Model file for the job. Use its own axes, mm. Face numbers are marked on the shaded views. A direction names the side the tool comes from. Round coordinates to 2 decimals unless told otherwise and drop trailing zeros. Write each loop counter-clockwise with the first axis right and the second up, starting at its lowest first coordinate (ties: lowest second). Pieces come first, ordered by that corner, then holes. Notation, with made-up numbers: (80.25, 69) - (105.25, 69) arc R26 cw to (105.25, 91) - close; hole circle Ø1 at (4.5, 71). An arc over 180 degrees is marked (long way). One line per item, written item: value.
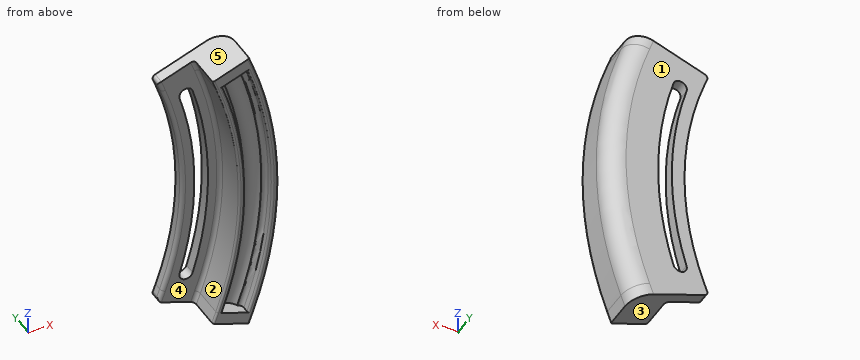
from build123d import *

# Parameters (mm, degrees)
REVOLVE_1_ANGLE     = 40
CUT_EXTRUDE_1_DEPTH = 10
FILLET_1_R          = 5
FILLET_3_R          = 1
FILLET_4_R          = 1
EXTRUDE_1_DEPTH     = 3
EXTRUDE_2_DEPTH     = 3
FILLET_6_R          = 0.5
FILLET_7_R          = 1


with BuildPart() as part:
    # 草图2 → 旋转1 (revolve, symmetric)
    with BuildSketch(Plane.XY) as revolve_1_sk:
        with BuildLine():
            Line((95, 4), (95, -5))
            Line((95, -5), (96.5, -5))
            Line((96.5, -5), (96.5, -2))
            Line((96.5, -2), (97.763932023, -2))
            ThreePointArc((97.763932023, -2), (100, -1), (102.236067977, -2))
            Line((102.236067977, -2), (103.5, -2))
            Line((103.5, -2), (103.5, -5))
            Line((103.5, -5), (105, -5))
            Line((105, -5), (105, 7))
            Line((105, 7), (85, 7))
            Line((85, 7), (85, 4))
            Line((85, 4), (95, 4))
        make_face()
    revolve(axis=Axis((0, 24.366902053, 0), (0, -1, 0)), revolution_arc=REVOLVE_1_ANGLE / 2)
    revolve(revolve_1_sk.sketch, axis=Axis((0, 24.366902053, 0), (0, 1, 0)), revolution_arc=REVOLVE_1_ANGLE / 2)

    # 草图3 → 切除-拉伸1 (cut)
    with BuildSketch(Plane(origin=(0, 7, 0), x_dir=(1, 0, 0), z_dir=(0, 1, 0))):
        with BuildLine():
            ThreePointArc((87.826997293, -26.542061834), (91.75, 1.18e-07), (87.826997225, 26.542062061))
            ThreePointArc((87.826997225, 26.542062061), (85.645571172, 27.710984674), (84.476648452, 25.529558679))
            ThreePointArc((84.476648452, 25.529558679), (88.25, 3.69e-07), (84.476648665, -25.529557973))
            ThreePointArc((84.476648665, -25.529557973), (85.645570933, -27.710984602), (87.826997293, -26.542061834))
        make_face()
    extrude(amount=-CUT_EXTRUDE_1_DEPTH, mode=Mode.SUBTRACT)

    # 圆角1
    fillet_1_edges = [part.edges().sort_by_distance(p)[0] for p in [
        (105, 7, 0),
    ]]
    fillet(fillet_1_edges, radius=FILLET_1_R)

    # 圆角3
    fillet_3_edges = [part.edges().sort_by_distance(p)[0] for p in [
        (95, 4, 0),
    ]]
    fillet(fillet_3_edges, radius=FILLET_3_R)

    # 圆角4
    fillet_4_edges = [part.edges().sort_by_distance(p)[0] for p in [
        (103.5, -2, 0),
        (96.5, -2, 0),
    ]]
    fillet(fillet_4_edges, radius=FILLET_4_R)

    # 草图5 → 凸台-拉伸1 (add)
    with BuildSketch(Plane(origin=(0, 0, 0), x_dir=(0.9396926207859081, 0, 0.34202014332566955), z_dir=(-0.34202014332566955, 0, 0.9396926207859082))):
        with BuildLine():
            Line((96.5, -5), (103.5, -5))
            Line((103.5, -5), (103.5, -3))
            ThreePointArc((103.5, -3), (103.207106781, -2.292893219), (102.5, -2))
            Line((102.5, -2), (102.236067977, -2))
            ThreePointArc((102.236067977, -2), (100, -1), (97.763932023, -2))
            Line((97.763932023, -2), (97.5, -2))
            ThreePointArc((97.5, -2), (96.792893219, -2.292893219), (96.5, -3))
            Line((96.5, -3), (96.5, -5))
        make_face()
        with BuildLine():
            Line((103.5, -5), (105, -5))
            Line((105, -5), (105, 2))
            ThreePointArc((105, 2), (103.535533906, 5.535533906), (100, 7))
            Line((100, 7), (85, 7))
            Line((85, 7), (85, 4))
            Line((85, 4), (94, 4))
            ThreePointArc((94, 4), (94.707106781, 3.707106781), (95, 3))
            Line((95, 3), (95, -5))
            Line((95, -5), (96.5, -5))
            Line((96.5, -5), (96.5, -3))
            ThreePointArc((96.5, -3), (96.792893219, -2.292893219), (97.5, -2))
            Line((97.5, -2), (97.763932023, -2))
            ThreePointArc((97.763932023, -2), (100, -1), (102.236067977, -2))
            Line((102.236067977, -2), (102.5, -2))
            ThreePointArc((102.5, -2), (103.207106781, -2.292893219), (103.5, -3))
            Line((103.5, -3), (103.5, -5))
        make_face()
    extrude(amount=EXTRUDE_1_DEPTH)

    # 草图6 → 凸台-拉伸2 (add)
    with BuildSketch(Plane(origin=(0, 0, 0), x_dir=(-0.9396926207859082, 0, 0.34202014332566943), z_dir=(-0.34202014332566943, 0, -0.9396926207859082))):
        with BuildLine():
            Line((-103.5, -5), (-96.5, -5))
            Line((-96.5, -5), (-96.5, -3))
            ThreePointArc((-96.5, -3), (-96.792893219, -2.292893219), (-97.5, -2))
            Line((-97.5, -2), (-97.763932023, -2))
            ThreePointArc((-97.763932023, -2), (-100, -1), (-102.236067977, -2))
            Line((-102.236067977, -2), (-102.5, -2))
            ThreePointArc((-102.5, -2), (-103.207106781, -2.292893219), (-103.5, -3))
            Line((-103.5, -3), (-103.5, -5))
        make_face()
        with BuildLine():
            Line((-85, 4), (-85, 7))
            Line((-85, 7), (-100, 7))
            ThreePointArc((-100, 7), (-103.535533906, 5.535533906), (-105, 2))
            Line((-105, 2), (-105, -5))
            Line((-105, -5), (-103.5, -5))
            Line((-103.5, -5), (-103.5, -3))
            ThreePointArc((-103.5, -3), (-103.207106781, -2.292893219), (-102.5, -2))
            Line((-102.5, -2), (-102.236067977, -2))
            ThreePointArc((-102.236067977, -2), (-100, -1), (-97.763932023, -2))
            Line((-97.763932023, -2), (-97.5, -2))
            ThreePointArc((-97.5, -2), (-96.792893219, -2.292893219), (-96.5, -3))
            Line((-96.5, -3), (-96.5, -5))
            Line((-96.5, -5), (-95, -5))
            Line((-95, -5), (-95, 3))
            ThreePointArc((-95, 3), (-94.707106781, 3.707106781), (-94, 4))
            Line((-94, 4), (-85, 4))
        make_face()
    extrude(amount=EXTRUDE_2_DEPTH)

    # 圆角6
    fillet_6_edges = [part.edges().sort_by_distance(p)[0] for p in [
        (88.75776876, -5, 33.901452547),
        (98.154694968, -5, 37.32165398),
        (98.154694968, -5, -37.32165398),
        (88.75776876, -5, -33.901452547),
        (105, -5, 0),
        (103.5, -5, 0),
        (96.5, -5, 0),
        (95, -5, 0),
    ]]
    fillet(fillet_6_edges, radius=FILLET_6_R)

    # 圆角7
    fillet_7_edges = [part.edges().sort_by_distance(p)[0] for p in [
        (79.360842552, 4, 30.481251114),
        (78.847812337, 5.5, 31.890790045),
        (79.360842552, 4, -30.481251114),
        (78.847812337, 5.5, -31.890790045),
        (85, 4, 0),
    ]]
    fillet(fillet_7_edges, radius=FILLET_7_R)


solid = part.part
1. Band-saw the part on B-B on y = 0.75. Write the cut outline in (x, z).
Report:
outline: (88.24, -35.31) - (97.64, -38.73) - (98.67, -35.91) arc R105 ccw to (98.67, 35.91) - (97.64, 38.73) - (88.24, 35.31) - (89.27, 32.49) arc R95 cw to (89.27, -32.49) - close
2. Mould opens along Z. For the marked faces 3, 4 and 5 say: released by +Z, released by -Z, zero draft, split by the parting line, or undercut.
Report:
face 3: released by -Z
face 4: undercut
face 5: released by +Z
3. Drop flat-ended pins along their axis: pin 1 (1.9 mm diameter, centred on x = 99, z = -14.5, fed in from -Y); pin 2 (1 mm diameter, centred on y = 5.5, z = -26, fed in from -X); pin 3 (1.5 mm diameter, centred on y = 2.5, z = -30.5, fed in from +X). Give the stop position or say it passes through.
Report:
pin 1: y = -1.17
pin 2: x = 80.76
pin 3: x = 100.68
4. Wall check: probe 1 along Y at (x, z) = (86, 13.5); probe 2 along X at (y, z) = (6.25, 10.5); probe 3 along X at (y, z) = (-3.25, -18). Give the ranges that are in metal, low to high. Write a range as [from, to].
Report:
probe 1: [4, 7]
probe 2: [84.35, 87.62], [91.15, 102.1]
probe 3: [93.28, 94.81], [101.92, 103.45]
5. Band-saw the part on A-A on y = -3.75. Write the cut outline in (x, z), plus the area to 3 significant figures.
Report:
outline: (88.24, -35.31) - (97.64, -38.73) - (98.67, -35.91) arc R105 ccw to (98.67, 35.91) - (97.64, 38.73) - (88.24, 35.31) - (89.27, 32.49) arc R95 cw to (89.27, -32.49) - close; hole (90.68, -33) - (97.26, -35.4) arc R103.5 ccw to (97.26, 35.4) - (90.68, 33) arc R96.5 cw to start
area: 269 mm²
6. Tool access for the marked faces 1 and 2: list every direction of +Z, -Z, +X, -X, +Y, -Y with a clear straight run to the whole face (end or side of a thin tool).
Report:
face 1: +Z, -Z, +X, -X, +Y
face 2: -X, -Y
